Build history of the part. All positions in model axes, mm. Face numbers are marked on the shaded views. Give positions to 0.01 mm unless a question says otherwise; leave off trailing zeros. Loops run counter-clockwise (first coordinate to the right, second up) from the corner with the lowest first, then second, coordinate; pieces in that order, holes last. Notation, with made-up numbers: (20.5, -22) - (48.5, -22) arc R31 cw to (48.5, 15) - close; hole circle Ø4 at (55.25, 73.25). An arc over 180 degrees is marked (long way). Return JSON: item names as keys, results as strings. Group by question number.
1) Drop flat-ended pins along their axis: pin 1 (3 mm diameter, centred on y = -10, z = 114, fed in from -X); pin 2 (2 mm diameter, centred on y = -98.5, z = 172, fed in from +X); pin 3 (1.5 mm diameter, centred on y = -89, z = 118, fed in from +X). Give the stop position or say it passes through.
2) Slice it at C-C (z = 251). List the corners of the cut face in (x, y), and give its area (3 significant figures).
3) Slice it at A-A (y = 0). List the corners of the cut face in (x, z).
4) Mould opens along X. For the marked faces 1 and 2 say: released by +X, released by -X, zero draft, split by the parting line, or undercut.
5) Drill centre lines: probe 1 along Y at (x, z) = (0, 214); probe 2 along Y at (x, z) = (-76, 246); probe 3 along X at (y, z) = (-74.5, 21.5). Where is each one in solid material? Low to high. Write a range as from..to.
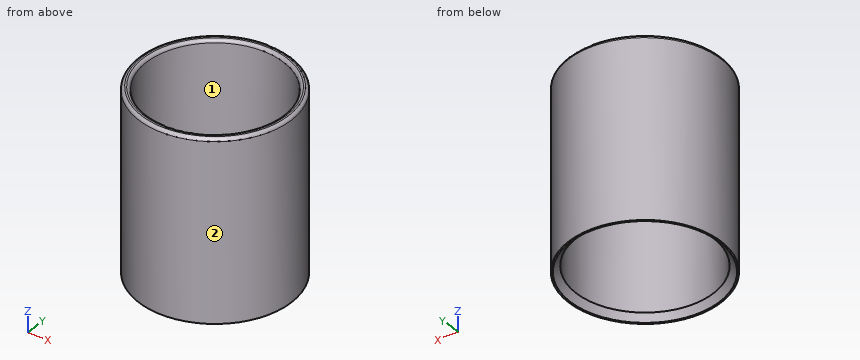
```python
from build123d import *

# Parameters (mm, degrees)
F0_R     = 127
F0_R_2   = 114.3
F1_DEPTH = 300
F2_R     = 5
F3_SIZE  = 10


with BuildPart() as f1:
    # F0 (on Top) → F1 (new body)
    with BuildSketch(Plane.XY):
        Circle(F0_R)
        Circle(F0_R_2, mode=Mode.SUBTRACT)
    extrude(amount=F1_DEPTH)

    # F2
    f2_edges = [f1.edges().sort_by_distance(p)[0] for p in [
        (-127, 0, 300),
        (-114.3, 0, 300),
    ]]
    fillet(f2_edges, radius=F2_R)

    # F3
    f3_edges = [f1.edges().sort_by_distance(p)[0] for p in [
        (-114.3, 0, 0),
    ]]
    chamfer(f3_edges, length=F3_SIZE)


solid = f1.part
```
Results:
{
 "1": {"pin 1": "x = -126.72", "pin 2": "x = 81.38", "pin 3": "x = 91.33"},
 "2": {"outline": "circle Ø254 at (0, 0); hole circle Ø228.6 at (0, 0)", "area": "9,630 mm2"},
 "3": {"outline": "(-127, 0) - (-124.3, 0) - (-114.3, 10) - (-114.3, 295) arc R5 ccw to (-119.3, 300) - (-122, 300) arc R5 ccw to (-127, 295) - close; (114.3, 10) - (124.3, 0) - (127, 0) - (127, 295) arc R5 ccw to (122, 300) - (119.3, 300) arc R5 ccw to (114.3, 295) - close"},
 "4": {"face 1": "undercut", "face 2": "split by the parting line"},
 "5": {"probe 1": "-127..-114.3, 114.3..127", "probe 2": "-101.75..-85.37, 85.37..101.75", "probe 3": "-102.85..-86.68, 86.68..102.85"}
}
